The model under review builds one solid part; all positions refer to its coordinate system, in mm. Give positions to 0.01 mm unless a question says otherwise; leave off trailing zeros. Order: outer loops, then holes, each group sorted by start corner. A loop starts at its lowest first (then second) coordinate and runs counter-clockwise, first axis right, second up. Notation, with made-up numbers: (6, -19) - (41, -19) arc R32 cw to (41, 19) - close; hole circle Ø1 at (15, 67). An arc over 180 degrees is marked (long way). Write item = value, one per line. Start each with the question number.
1. We need section A-A, the plane x = 133. Give the boundary of the cut face in (y, z).
2. Mouldability with a two-part tool opening along X and no side actions: class faces 1 (the flat face through (562, -16, 459)), 2 (the flat face through (76, -9, 463)) as pulls with the +X half, pulls with the -X half, needs draft (parallel to the pull), parting line crosses it, or undercut.
3. Wall thickness on probe 1 along Z at (x, y) = (210.5, -9.25); probe 2 along X at (y, z) = (-9.75, 668); probe 3 along Z at (x, y) = (472, -13.75): over which ranges is each line inside the solid? List them lowest first.
4. We need section B-B, the plane z = 485. Give the boundary of the cut face in (x, y).
from build123d import *

# Parameters (mm, degrees)
F0_W      = 44.656470418
F0_H      = 33.8078811765
F1_DEPTH  = 16
F2_DEPTH  = 796
F3_DEPTH  = 196
F4_W      = 68.9578056335
F4_H      = 493.6993122101
F5_DEPTH  = 7
F6_DEPTH  = 9.7
F7_DEPTH  = 99.33
F8_DEPTH  = 99.33
F9_DEPTH  = 17.34
F10_DEPTH = 102.97
F11_W     = 35.2807044983
F11_H     = 492.0964837074
F12_DEPTH = 7
F13_DEPTH = 37.27
F14_DEPTH = 6.58
F15_DEPTH = 106.63
F16_DEPTH = 5.87
F17_DEPTH = 200
F18_DEPTH = 200
F19_DEPTH = 200
F20_DEPTH = 200
F21_DEPTH = 200
F22_DEPTH = 200
F23_DEPTH = 200
F24_DEPTH = 200
F25_DEPTH = 200
F26_R     = 3


with BuildPart() as f1:
    # F0 (on Front) → F1 (new body)
    with BuildSketch(Plane.XZ):
        with Locations((22.328235209, 16.9039405882)):
            Rectangle(F0_W, F0_H)
    extrude(amount=F1_DEPTH)

    # F2 (add): a face of the model
    f2_faces = [f1.faces().sort_by_distance(p)[0] for p in [
        (22.328235209, -8, 0),
    ]]
    extrude(f2_faces, amount=-F2_DEPTH)

    # F3 (add): a face of the model
    f3_faces = [f1.faces().sort_by_distance(p)[0] for p in [
        (0, -8, 398),
    ]]
    extrude(f3_faces, amount=-F3_DEPTH)

    # F4 (on face) → F5 (cut)
    with BuildSketch(Plane.XZ.offset(16)):
        with Locations((94.1769480705, 399.8196721077)):
            Rectangle(F4_W, F4_H)
    extrude(amount=-F5_DEPTH, mode=Mode.SUBTRACT)

    # F6 (cut): a face of the model
    f6_faces = [f1.faces().sort_by_distance(p)[0] for p in [
        (59.6980452538, -12.5, 399.8196721077),
    ]]
    extrude(f6_faces, amount=-F6_DEPTH, mode=Mode.SUBTRACT)

    # F7 (add): a face of the model
    f7_faces = [f1.faces().sort_by_distance(p)[0] for p in [
        (89.3269480705, -12.5, 646.6693282127),
    ]]
    extrude(f7_faces, amount=-F7_DEPTH)

    # F8 (cut): a face of the model
    f8_faces = [f1.faces().sort_by_distance(p)[0] for p in [
        (89.3269480705, -12.5, 646.6693282127),
    ]]
    extrude(f8_faces, amount=-F8_DEPTH, mode=Mode.SUBTRACT)

    # F9 (cut): a face of the model
    f9_faces = [f1.faces().sort_by_distance(p)[0] for p in [
        (128.6558508873, -12.5, 449.4846721077),
    ]]
    extrude(f9_faces, amount=-F9_DEPTH, mode=Mode.SUBTRACT)

    # F10 (cut): a face of the model
    f10_faces = [f1.faces().sort_by_distance(p)[0] for p in [
        (97.9969480705, -12.5, 152.9700160027),
    ]]
    extrude(f10_faces, amount=-F10_DEPTH, mode=Mode.SUBTRACT)

    # F11 (on face) → F12 (join)
    with BuildSketch(Plane.XZ.offset(9)):
        with Locations((91.7714834213, 432.6795041561)):
            Rectangle(F11_W, F11_H)
    extrude(amount=F12_DEPTH)

    # F13 (add): a face of the model
    f13_faces = [f1.faces().sort_by_distance(p)[0] for p in [
        (91.7714834213, -12.5, 678.7277460098),
    ]]
    extrude(f13_faces, amount=F13_DEPTH)

    # F14 (add): a face of the model
    f14_faces = [f1.faces().sort_by_distance(p)[0] for p in [
        (109.4118356705, -12.5, 451.3145041561),
    ]]
    extrude(f14_faces, amount=F14_DEPTH)

    # F15 (add): a face of the model
    f15_faces = [f1.faces().sort_by_distance(p)[0] for p in [
        (95.0614834213, -12.5, 186.6312623024),
    ]]
    extrude(f15_faces, amount=F15_DEPTH)

    # F16 (cut): a face of the model
    f16_faces = [f1.faces().sort_by_distance(p)[0] for p in [
        (74.1311311722, -12.5, 397.9995041561),
    ]]
    extrude(f16_faces, amount=-F16_DEPTH, mode=Mode.SUBTRACT)

    # F17 (add): a face of the model
    f17_faces = [f1.faces().sort_by_distance(p)[0] for p in [
        (196, -8, 398),
    ]]
    extrude(f17_faces, amount=F17_DEPTH)

    # F18 (cut): a face of the model
    f18_faces = [f1.faces().sort_by_distance(p)[0] for p in [
        (145.9958508873, -12.5, 397.9996721077),
    ]]
    extrude(f18_faces, amount=-F18_DEPTH, mode=Mode.SUBTRACT)

    # F19 (add): a face of the model
    f19_faces = [f1.faces().sort_by_distance(p)[0] for p in [
        (115.9918356705, -12.5, 397.9995041561),
    ]]
    extrude(f19_faces, amount=F19_DEPTH)

    # F20 (add): a face of the model
    f20_faces = [f1.faces().sort_by_distance(p)[0] for p in [
        (396, -8, 398),
    ]]
    extrude(f20_faces, amount=F20_DEPTH)

    # F21 (cut): a face of the model
    f21_faces = [f1.faces().sort_by_distance(p)[0] for p in [
        (345.9958508873, -12.5, 397.9996721077),
    ]]
    extrude(f21_faces, amount=-F21_DEPTH, mode=Mode.SUBTRACT)

    # F22 (add): a face of the model
    f22_faces = [f1.faces().sort_by_distance(p)[0] for p in [
        (315.9918356705, -12.5, 397.9995041561),
    ]]
    extrude(f22_faces, amount=F22_DEPTH)

    # F23 (add): a face of the model
    f23_faces = [f1.faces().sort_by_distance(p)[0] for p in [
        (298, -8, 796),
    ]]
    extrude(f23_faces, amount=F23_DEPTH)

    # F24 (cut): a face of the model
    f24_faces = [f1.faces().sort_by_distance(p)[0] for p in [
        (297.9969480705, -12.5, 745.9993282127),
    ]]
    extrude(f24_faces, amount=-F24_DEPTH, mode=Mode.SUBTRACT)

    # F25 (add): a face of the model
    f25_faces = [f1.faces().sort_by_distance(p)[0] for p in [
        (297.9964834213, -12.5, 715.9977460098),
    ]]
    extrude(f25_faces, amount=F25_DEPTH)

    # F26
    f26_edges = [f1.edges().sort_by_distance(p)[0] for p in [
        (0, -16, 498),
        (298, -16, 0),
        (596, -16, 498),
        (298, -16, 996),
        (297.996948, -16, 50.000016),
        (49.998045, -16, 497.999672),
        (297.996948, -16, 945.999328),
        (545.995851, -16, 497.999672),
        (80.001131, -16, 497.999504),
        (297.996483, -16, 80.001262),
        (515.991836, -16, 497.999504),
        (297.996483, -16, 915.997746),
    ]]
    fillet(f26_edges, radius=F26_R)


solid = f1.part
Model answer:
q1.outline = (-16, 3) arc R3 ccw to (-13, 0) - (0, 0) - (0, 996) - (-13, 996) arc R3 ccw to (-16, 993) - (-16, 949) arc R3 ccw to (-13, 946) - (-9, 946) - (-9, 916) - (-13, 916) arc R3 ccw to (-16, 913) - (-16, 83) arc R3 ccw to (-13, 80) - (-9, 80) - (-9, 50) - (-13, 50) arc R3 ccw to (-16, 47) - close
q2.face_1 = needs draft
q2.face_2 = undercut
q3.probe_1 = 0 to 50, 80 to 916, 946 to 996
q3.probe_2 = 0 to 50, 80 to 515.99, 546 to 596
q3.probe_3 = 0.1 to 49.9, 80.1 to 915.9, 946.09 to 995.9
q4.outline = (0, -13) arc R3 ccw to (3, -16) - (47, -16) arc R3 ccw to (50, -13) - (50, -9) - (80, -9) - (80, -13) arc R3 ccw to (83, -16) - (512.99, -16) arc R3 ccw to (515.99, -13) - (515.99, -9) - (546, -9) - (546, -13) arc R3 ccw to (549, -16) - (593, -16) arc R3 ccw to (596, -13) - (596, 0) - (0, 0) - close
